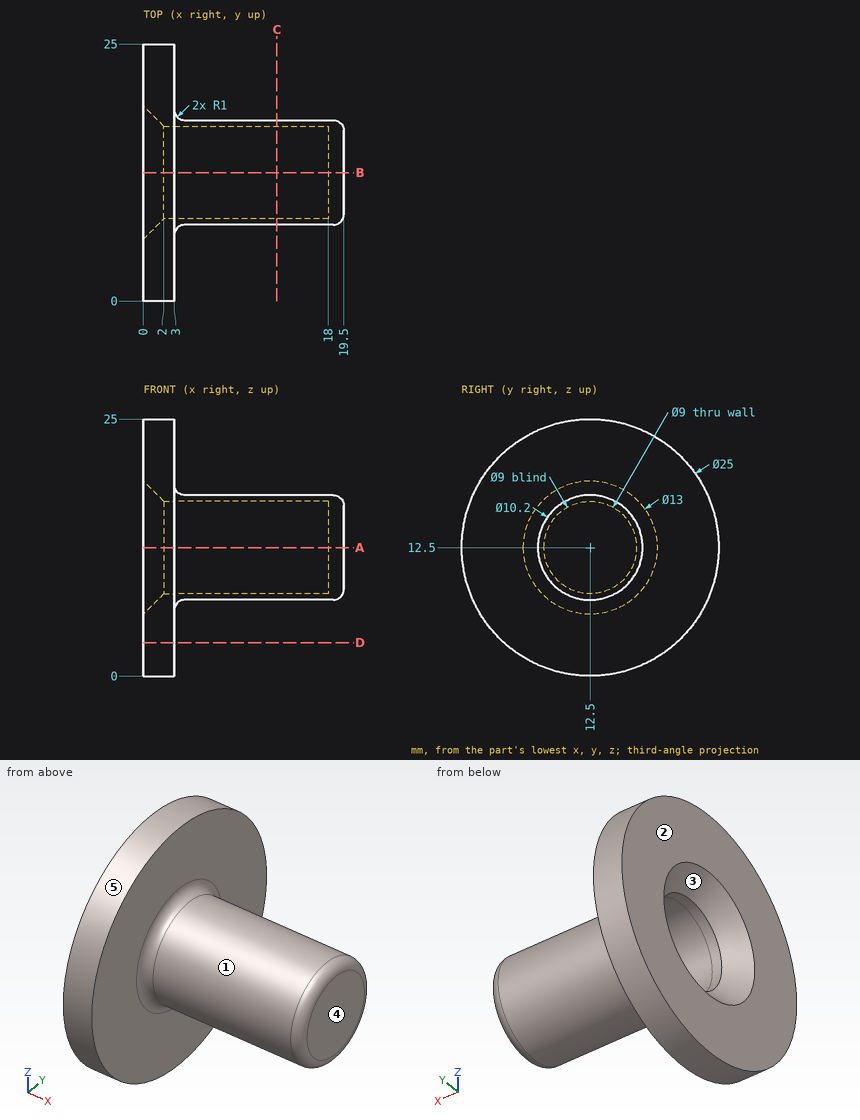
The drawing under review shows one solid part. Ordinate dimensions are in mm from its lowest x, y, z. A direction names the side the tool comes from. Coordinates: 2 decimals unless noted, no trailing zeros. Loops run counter-clockwise (first coordinate to the right, second up) from the corner with the lowest first, then second, coordinate; pieces in that order, holes last. Notation, with made-up numbers: (50.25, 32) - (68.25, 32) arc R21 cw to (68.25, 45) - close; hole circle Ø5 at (-33, -37.75). An arc over 180 degrees is marked (long way). Return JSON: item names as keys, results as strings.
Item 1: Take a section at D-D (z = 3.25). Give the boundary of the cut face in (x, y).
Determined:
{"outline": "(0, 4.09) - (3, 4.09) - (3, 20.91) - (0, 20.91) - close"}
Item 2: Take a section at C-C (x = 13). Give the boundary of the cut face in (y, z), then the cut area to 3 significant figures.
Determined:
{"outline": "circle Ø10.2 at (12.5, 12.5); hole circle Ø9 at (12.5, 12.5)", "area": "18.1 mm2"}
Item 3: Insertion check: pin 1 (5.5 mm diameter, centred on y = 12.5, z = 12.5, fed in from -X); pin 2 (2 mm diameter, centred on y = 6.5, z = 5, fed in from +X); pin 3 (10 mm diameter, centred on x = 5.5, y = 5.5, fed in from +Z); pin 4 (1 mm diameter, centred on x = 11, y = 20, fed in from -Z). Each pin has a flat end and moves straight along its axis. Give the tip position at first contact, or say it passes through.
Determined:
{"pin 1": "stops at x = 18", "pin 2": "stops at x = 3", "pin 3": "stops at z = 24.71", "pin 4": "passes through"}
Item 4: Mouldability with a two-part tool opening along Y and no side actions: class the marked faces 3, 4 and 5 as pulls with the +Y half, pulls with the -Y half, needs draft (parallel to the pull), parting line crosses it, or undercut.
Determined:
{"face 3": "undercut", "face 4": "needs draft", "face 5": "parting line crosses it"}
Item 5: For the marked faces 1 and 2, list the 3-axis set-ups (+Z, -Z, +X, -X, +Y, -Y) from which the entire face can be reached by the end or side of a thin tool; tool diameter is ignored.
Determined:
{"face 1": "+X", "face 2": "+Z, -Z, -X, +Y, -Y"}
Item 6: For line 1 (Z direction, x = 9.5, y = 12.5); line 2 (Z direction, x = 2.5, y = 12.5); line 3 (X direction, y = 6.25, z = 3.5), list the stretches that pass through material, from the lowest coordinate up.
Determined:
{"line 1": "z = 7.4 to 8, 17 to 17.6", "line 2": "z = 0 to 8, 17 to 25", "line 3": "x = 0 to 3"}
Item 7: Take a section at A-A (z = 12.5). Give the boundary of the cut face in (x, y).
Determined:
{"outline": "(0, 0) - (3, 0) - (3, 6.4) arc R1 cw to (4, 7.4) - (18.5, 7.4) arc R1 ccw to (19.5, 8.4) - (19.5, 16.6) arc R1 ccw to (18.5, 17.6) - (4, 17.6) arc R1 cw to (3, 18.6) - (3, 25) - (0, 25) - (0, 19) - (2, 17) - (18, 17) - (18, 8) - (2, 8) - (0, 6) - close"}
